from build123d import *

# Parameters (mm, degrees)
F0_W     = 20
F0_H     = 20
F0_R     = 0.18
F1_DEPTH = 20
F4_R     = 2.5
F2_W     = 10
F2_H     = 10
F6_R     = 0.18


with BuildPart() as f1:
    # F0 (on Top) → F1 (new body)
    with BuildSketch(Plane.XY):
        Rectangle(F0_W, F0_H)
        Circle(F0_R, mode=Mode.SUBTRACT)
    extrude(amount=F1_DEPTH)

    # F4 (on offset) → F7 section 0
    with BuildSketch(Plane.XY.offset(15)):
        Circle(F4_R)
    # F2 (on face) → F7 section 1
    with BuildSketch(Plane.XY.offset(20)):
        Rectangle(F2_W, F2_H)
    loft(mode=Mode.SUBTRACT)

    # F4 (on offset) → F8 section 0
    with BuildSketch(Plane.XY.offset(15)):
        Circle(F4_R)
    # F6 (on offset) → F8 section 1
    with BuildSketch(Plane.XY.offset(5)):
        Circle(F6_R)
    loft(mode=Mode.SUBTRACT)

    # F10 (on offset) → F11 (revolve, cut)
    with BuildSketch(Plane(origin=(0, 0, 0), x_dir=(0, -1, 0), z_dir=(-1, 0, 0))):
        Polygon((0.4, 0), (0, 1), (0, 0), align=None)
    revolve(axis=Axis((0, 0, 0.5), (0, 0, 1)), mode=Mode.SUBTRACT)


solid = f1.part
The model under review builds one solid part; all positions refer to its coordinate system, in mm. Give positions to 0.01 mm unless a question says otherwise; leave off trailing zeros. Loops run counter-clockwise (first coordinate to the right, second up) from the corner with the lowest first, then second, coordinate; pieces in that order, holes last. Notation, with made-up numbers: (60.25, 63.5) -> (68.25, 63.5) arc R17 ccw to (68.25, 89.5) -> close; hole circle Ø9 at (39.25, 18.5). An arc over 180 degrees is marked (long way). Answer as a JSON object with one key per item and string values. Group by question number.
Q1. Take a section at A-A (z = 13.5). Write out the cut boundary in (x, y), plus the area to 3 significant figures.
Q2. Wall thickness on line 1 along X through (y, z) = (0, 2); line 2 along Y through (x, z) = (-0.25, 6.5): over which ranges is each line inside the solid? List them lowest first.
Q3. Draft analysis for pull direction Y (two halves, no side actions). For faces 1 (the flat face through (-10, 0, 10)), 2 (the flat face through (0, -10, 10)), 3 (the conical face through (0.712, 1.116, 9.93)), state which applies: pulls with the +Y half, pulls with the -Y half, needs draft (parallel to the pull), parting line crosses it, or undercut.
Answer below:
{
 "1": {"outline": "(-10, -10) -> (10, -10) -> (10, 10) -> (-10, 10) -> close; hole circle Ø4.3 at (0, 0)", "area": "385 mm2"},
 "2": {"line 1": "x = -10 to -0.18, 0.18 to 10", "line 2": "y = -10 to -0.47, 0.47 to 10"},
 "3": {"face 1": "needs draft", "face 2": "pulls with the -Y half", "face 3": "undercut"}
}
